Build history of the part. All positions in model axes, mm. Face numbers are marked on the shaded views. A direction names the side the tool comes from. Give positions to 0.01 mm unless a question says otherwise; leave off trailing zeros. Order: outer loops, then holes, each group sorted by start corner. A loop starts at its lowest first (then second) coordinate and runs counter-clockwise, first axis right, second up. Notation, with made-up numbers: (-25.75, 70.5) - (-21.75, 70.5) arc R8 ccw to (-21.75, 77.5) - close; hole circle Ø7 at (-7, 51). An arc over 180 degrees is marked (long way). Use a Markdown table: item, result. Add a question column.
(1) Slice it at B-B (x = -11). Write the cut outline in (y, z), then the cut area to 3 significant figures.
(2) Slice it at C-C (z = 283). Write the cut outline in (x, y).
(3) Slice it at D-D (x = 170.5). Write the cut outline in (y, z), then the cut area to 3 significant figures.
(4) Wall check: line 1 (X direction, y = 264.5, z = 156.5); line 2 (Z direction, x = 105, y = 289); line 3 (X direction, y = 299, z = 207.5). Give the ranges that are in metal, low to high.
(5) Mould opens along Z. For the marked faces 1, 2 and 3 say: +Z half, -Z half, draft (parallel to the pull), parting line (faces both ways), or undercut.
(6) Which spindle directions (+Z, -Z, +X, -X, +Y, -Y) get a long thin tool onto all of the face, cutting with end or side? Do the marked faces 4, 5, 6, 7 and 8. Say none if no direction does.
(7) Flat gauge pins, fed straight in: pin 1 (4 mm diameter, centred on x = 51.5, z = 118, fed in from +Y); pin 2 (1 mm diameter, centred on x = 147, z = 202.5, fed in from +Y); pin 3 (1.5 mm diameter, centred on x = 31, z = 317.5, fed in from -Y). Where does each tip first touch, or does it go through?
(8) Slice it at A-A (y = 286.5). Write the cut outline in (x, z), then the cut area to 3 significant figures.
from build123d import *

# Parameters (mm, degrees)
BOSS_EXTRUDE1_DEPTH = 320
SKETCH2_W           = 20
SKETCH2_H           = 20
BOSS_EXTRUDE2_DEPTH = 5
SKETCH3_W           = 15
SKETCH3_H           = 15
BOSS_EXTRUDE3_DEPTH = 5
SKETCH4_W           = 10
SKETCH4_H           = 10
BOSS_EXTRUDE4_DEPTH = 20
BOSS_EXTRUDE5_REACH = 232.496
SKETCH5_W           = 10
SKETCH5_H           = 10
SKETCH6_W           = 290
SKETCH6_H           = 280
CUT_EXTRUDE1_DEPTH  = 120
SKETCH7_W           = 360
SKETCH7_H           = 135
BOSS_EXTRUDE6_DEPTH = 5
SKETCH8_W           = 370
SKETCH8_H           = 145
BOSS_EXTRUDE7_DEPTH = 5
SKETCH9_W           = 380
SKETCH9_H           = 155
BOSS_EXTRUDE8_DEPTH = 5
SKETCH10_W          = 390
SKETCH10_H          = 165
BOSS_EXTRUDE9_DEPTH = 5


with BuildPart() as part:
    # Sketch1 → Boss-Extrude1 (new body)
    with BuildSketch(Plane.XY):
        Polygon((-175, 206.36092205), (175, 206.36092205), (175, 258.86092205), (155, 258.86092205), (155, 278.86092205), (175, 278.86092205), (175, 331.36092205), (-175, 331.36092205), (-175, 278.86092205), (-155, 278.86092205), (-155, 258.86092205), (-175, 258.86092205), align=None)
    extrude(amount=BOSS_EXTRUDE1_DEPTH)

    # Sketch2 → Boss-Extrude2 (add)
    with BuildSketch(Plane.XY.offset(320)):
        with Locations((60, 268.86092205)):
            Rectangle(SKETCH2_W, SKETCH2_H)
        with Locations((-60, 268.86092205)):
            Rectangle(SKETCH2_W, SKETCH2_H)
    extrude(amount=BOSS_EXTRUDE2_DEPTH)

    # Sketch3 → Boss-Extrude3 (add)
    with BuildSketch(Plane.XY.offset(325)):
        with Locations((60, 268.86092205)):
            Rectangle(SKETCH3_W, SKETCH3_H)
        with Locations((-60, 268.86092205)):
            Rectangle(SKETCH3_W, SKETCH3_H)
    extrude(amount=BOSS_EXTRUDE3_DEPTH)

    # Sketch4 → Boss-Extrude4 (add)
    with BuildSketch(Plane.XY.offset(330)):
        with Locations((60.496067434, 268.65644762)):
            Rectangle(SKETCH4_W, SKETCH4_H)
        with Locations((-60.496067434, 268.65644762)):
            Rectangle(SKETCH4_W, SKETCH4_H)
    extrude(amount=BOSS_EXTRUDE4_DEPTH)

    # Sketch5 → Boss-Extrude5 (add, up to next)
    with BuildSketch(Plane.ZY.offset(-55.496067434), mode=Mode.PRIVATE) as boss_extrude5_sk1:
        with Locations((345, 268.65644762)):
            Rectangle(SKETCH5_W, SKETCH5_H)
    boss_extrude5_tool1 = extrude(boss_extrude5_sk1.sketch, amount=BOSS_EXTRUDE5_REACH, mode=Mode.PRIVATE) - part.part
    add(boss_extrude5_tool1.solids().sort_by_distance((55.496067, 268.656448, 345))[0])

    # Sketch6 → Cut-Extrude1 (cut)
    with BuildSketch(Plane(origin=(0, 331.36092205, 0), x_dir=(1, 0, 0), z_dir=(0, 1, 0))):
        with Locations((0, -160)):
            Rectangle(SKETCH6_W, SKETCH6_H)
    extrude(amount=-CUT_EXTRUDE1_DEPTH, mode=Mode.SUBTRACT)

    # Sketch7 → Boss-Extrude6 (add)
    with BuildSketch(Plane.XY.offset(320)):
        with Locations((0, 268.86092205)):
            Rectangle(SKETCH7_W, SKETCH7_H)
    extrude(amount=-BOSS_EXTRUDE6_DEPTH)

    # Sketch8 → Boss-Extrude7 (add)
    with BuildSketch(Plane(origin=(0, 0, 315), x_dir=(-1, 0, 0), z_dir=(0, 0, -1))):
        with Locations((0, 268.86092205)):
            Rectangle(SKETCH8_W, SKETCH8_H)
    extrude(amount=BOSS_EXTRUDE7_DEPTH)

    # Sketch9 → Boss-Extrude8 (add)
    with BuildSketch(Plane(origin=(0, 0, 310), x_dir=(-1, 0, 0), z_dir=(0, 0, -1))):
        with Locations((0, 268.86092205)):
            Rectangle(SKETCH9_W, SKETCH9_H)
    extrude(amount=BOSS_EXTRUDE8_DEPTH)

    # Sketch10 → Boss-Extrude9 (add)
    with BuildSketch(Plane(origin=(0, 0, 305), x_dir=(-1, 0, 0), z_dir=(0, 0, -1))):
        with Locations((0, 268.86092205)):
            Rectangle(SKETCH10_W, SKETCH10_H)
    extrude(amount=BOSS_EXTRUDE9_DEPTH)


solid = part.part
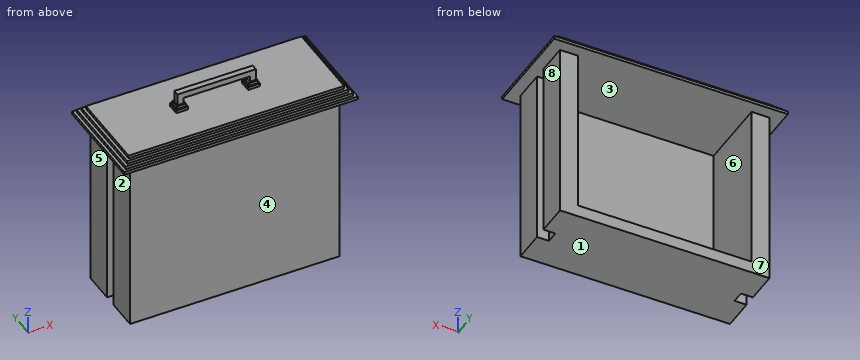
Solution:
| question | item | result |
|---|---|---|
| 1 | outline | (186.36, 300) - (206.36, 300) - (206.36, 0) - (331.36, 0) - (331.36, 20) - (211.36, 20) - (211.36, 300) - (351.36, 300) - (351.36, 305) - (346.36, 305) - (346.36, 310) - (341.36, 310) - (341.36, 315) - (336.36, 315) - (336.36, 320) - (201.36, 320) - (201.36, 315) - (196.36, 315) - (196.36, 310) - (191.36, 310) - (191.36, 305) - (186.36, 305) - close; (263.66, 340) - (273.66, 340) - (273.66, 350) - (263.66, 350) - close |
| 1 | area | 7,000 mm2 |
| 2 | outline | (-175, 206.36) - (175, 206.36) - (175, 258.86) - (155, 258.86) - (155, 278.86) - (175, 278.86) - (175, 331.36) - (145, 331.36) - (145, 211.36) - (-145, 211.36) - (-145, 331.36) - (-175, 331.36) - (-175, 278.86) - (-155, 278.86) - (-155, 258.86) - (-175, 258.86) - close |
| 3 | outline | (186.36, 300) - (206.36, 300) - (206.36, 0) - (258.86, 0) - (258.86, 300) - (278.86, 300) - (278.86, 0) - (331.36, 0) - (331.36, 300) - (351.36, 300) - (351.36, 305) - (346.36, 305) - (346.36, 310) - (341.36, 310) - (341.36, 315) - (336.36, 315) - (336.36, 320) - (201.36, 320) - (201.36, 315) - (196.36, 315) - (196.36, 310) - (191.36, 310) - (191.36, 305) - (186.36, 305) - close |
| 3 | area | 34,500 mm2 |
| 4 | line 1 | -155 to -145, 145 to 155 |
| 4 | line 2 | 0 to 20, 300 to 320 |
| 4 | line 3 | -175 to -145, 145 to 175 |
| 5 | face 1 | -Z half |
| 5 | face 2 | draft |
| 5 | face 3 | undercut |
| 6 | face 4 | -Z, +X, -X, -Y |
| 6 | face 5 | -Z, -X, +Y, -Y |
| 6 | face 6 | +Y |
| 6 | face 7 | -Z, +X, -X, +Y |
| 6 | face 8 | -Z, +X, +Y, -Y |
| 7 | pin 1 | y = 211.36 |
| 7 | pin 2 | y = 331.36 |
| 7 | pin 3 | y = 201.36 |
| 8 | outline | (-195, 300) - (-175, 300) - (-175, 0) - (175, 0) - (175, 300) - (195, 300) - (195, 305) - (190, 305) - (190, 310) - (185, 310) - (185, 315) - (180, 315) - (180, 320) - (-180, 320) - (-180, 315) - (-185, 315) - (-185, 310) - (-190, 310) - (-190, 305) - (-195, 305) - close; hole (-145, 20) - (145, 20) - (145, 300) - (-145, 300) - close |
| 8 | area | 31,300 mm2 |
